```python
from build123d import *

# Parameters (mm, degrees)
ESQUISSE1_W        = 34
ESQUISSE1_H        = 74
ESQUISSE1_W_2      = 30
ESQUISSE1_H_2      = 70
BOSS_EXTRU_1_DEPTH = 135
ESQUISSE1_2_W      = 34
ESQUISSE1_2_H      = 74
ESQUISSE1_2_W_2    = 30
ESQUISSE1_2_H_2    = 70
BOSS_EXTRU_2_DEPTH = 2


with BuildPart() as part:
    # Esquisse1 → Boss.-Extru.1 (new body)
    with BuildSketch(Plane(origin=(0, 0, 0), x_dir=(1, 0, 0), z_dir=(0, 1, 0))):
        Rectangle(ESQUISSE1_W, ESQUISSE1_H)
        Rectangle(ESQUISSE1_W_2, ESQUISSE1_H_2, mode=Mode.SUBTRACT)
    extrude(amount=BOSS_EXTRU_1_DEPTH)

    # Esquisse1_2 → Boss.-Extru.2 (add)
    with BuildSketch(Plane(origin=(0, 0, 0), x_dir=(1, 0, 0), z_dir=(0, 1, 0))):
        Rectangle(ESQUISSE1_2_W, ESQUISSE1_2_H)
        Rectangle(ESQUISSE1_2_W_2, ESQUISSE1_2_H_2, mode=Mode.SUBTRACT)
        Rectangle(ESQUISSE1_2_W_2, ESQUISSE1_2_H_2)
    extrude(amount=-BOSS_EXTRU_2_DEPTH)


solid = part.part
```
Model file for the job. Use its own axes, mm. A direction names the side the tool comes from. Give positions to 0.01 mm unless a question says otherwise; leave off trailing zeros. Loops run counter-clockwise (first coordinate to the right, second up) from the corner with the lowest first, then second, coordinate; pieces in that order, holes last. Notation, with made-up numbers: (-8, 1.25) -> (14, 1.25) arc R20 cw to (14, 36.25) -> close; hole circle Ø4 at (65, 37). An arc over 180 degrees is marked (long way). Use CSV: the item, a comma, the result in double quotes. Start each with the question number.
1) Slice it at C-C on x = 5.5. Give the cut face in (y, z), plus the area to 3 significant figures.
2) Slice it at B-B on y = 115. Give the cut face in (x, z), plus the area to 3 significant figures.
3) Tool access for faces 1 (the flat face through (-15.2, 135, -2.9)), 2 (the flat face through (15, 67, 0)): list every direction of +Z, -Z, +X, -X, +Y, -Y with a clear straight run to the whole face (end or side of a thin tool).
4) Slice it at A-A on z = 6.5. Give the cut face in (x, y).
5) Mould opens along Z. For faces 3 (the flat face through (0, 67, -35)), 4 (the flat face through (-17, 67, 1)), 5 (the flat face through (0, 67, -37)), 6 (the flat face through (0, 67, 37)) say: released by +Z, released by -Z, zero draft, split by the parting line, or undercut.
6) Wall check: line 1 (X direction, y = 25, z = 23); line 2 (Z direction, x = -2, y = 69.5); line 3 (Y direction, x = -9, z = 1.5). Give the ranges that are in metal, low to high.
Computed values:
1,outline,"(-2, -37) -> (135, -37) -> (135, -35) -> (0, -35) -> (0, 35) -> (135, 35) -> (135, 37) -> (-2, 37) -> close"
1,area,"688 mm^2"
2,outline,"(-17, -37) -> (17, -37) -> (17, 37) -> (-17, 37) -> close; hole (-15, -35) -> (15, -35) -> (15, 35) -> (-15, 35) -> close"
2,area,"416 mm^2"
3,face 1,"+Z, -Z, +X, -X, +Y"
3,face 2,"+Y"
4,outline,"(-17, -2) -> (17, -2) -> (17, 135) -> (15, 135) -> (15, 0) -> (-15, 0) -> (-15, 135) -> (-17, 135) -> close"
5,face 3,"undercut"
5,face 4,"zero draft"
5,face 5,"released by -Z"
5,face 6,"released by +Z"
6,line 1,"x = -17 to -15, 15 to 17"
6,line 2,"z = -37 to -35, 35 to 37"
6,line 3,"y = -2 to 0"
